Answer from the drawing. Dimensions are ordinates in mm from the lowest x, y and z of the part. A direction names the side the tool comes from. Give positions to 0.01 mm unless a question says otherwise; leave off trailing zeros. Loops run counter-clockwise (first coordinate to the right, second up) from the corner with the lowest first, then second, coordinate; pieces in that order, holes last. Notation, with made-up numbers: (17, -18) - (76, -18) arc R11 ccw to (76, 3) - close; hole circle Ø5 at (28, 10.5). An arc over 180 degrees is marked (long way). Write each question's results on one line, items separated by ' | '. Start each with the question number.
Q1. Given pin 1 (6.5 mm diameter, centred on x = 5, z = 7.5, fed in from +Y); pin 2 (4 mm diameter, centred on y = 2, z = 4, fed in from +X); pin 3 (4 mm diameter, centred on y = 12, z = 7, fed in from -X), each flat-ended and moving along its own axis, determine where each tip first touches the part or whether it passes through.
Q2. The part is cut by section B-B, the plane x = 7.62. Write down the section's boundary in (y, z) (1 decimal).
Q3. Determine the mould class of the marked faces 1, 2, 3 and 4 for opening direction Z: +Z half, -Z half, draft (parallel to the pull), parting line (faces both ways), or undercut.
Q4. The part is cut by section C-C, the plane z = 8.5. State how many separate pieces and enclosed holes the cut face has.
Q5. For the marked faces 5 and 6, determine the directions among +Z, -Z, +X, -X, +Y, -Y from which every point of the face is accessible in a straight line to the end or side of a thin tool.
Q6. Find the intervals of material crossed by line 1 (X direction, y = 13.25, z = 10); line 2 (Z direction, x = 7.62, y = 1.4) (1 decimal); line 3 (Y direction, x = 4, z = 1.5), in increasing order. Write a range as from..to.
Q7. The part is cut by section D-D, the plane y = 7.75. Write down the section's boundary in (x, z).
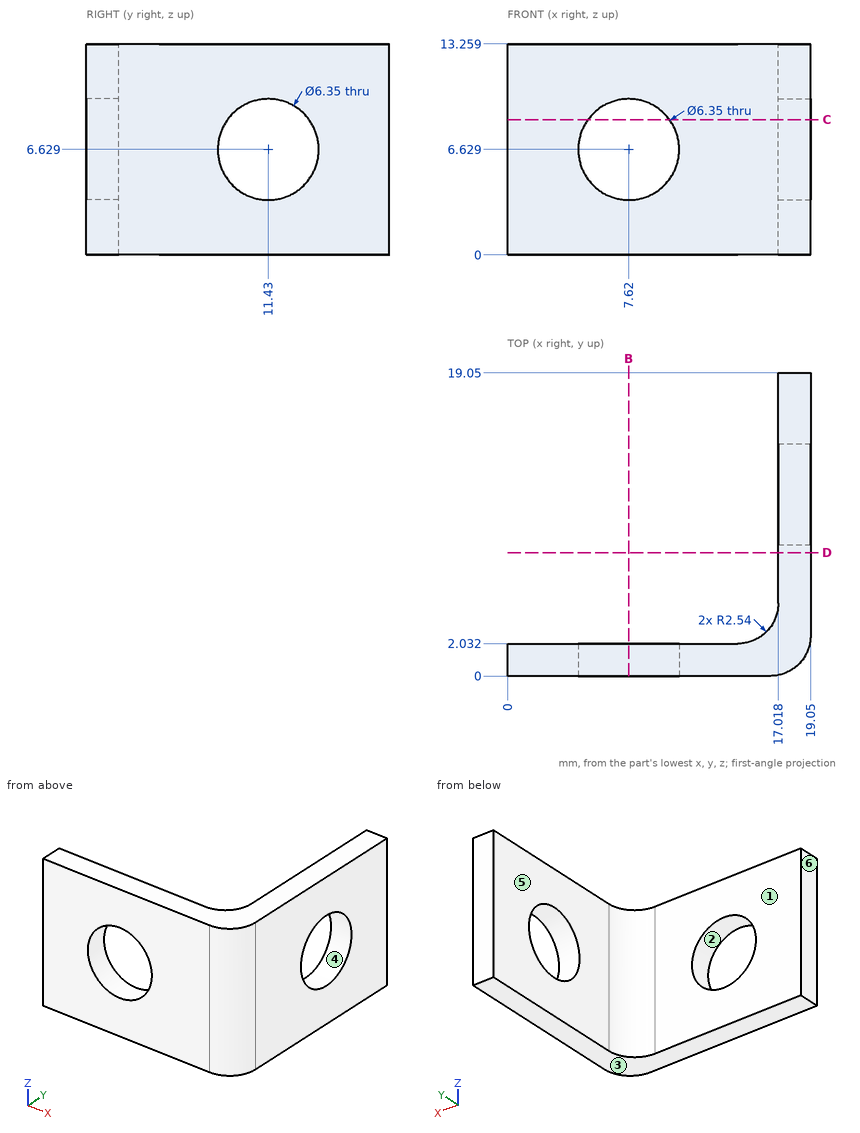
Check sheet entries:
1) pin 1: stops at y = 2.03 | pin 2: stops at x = 19.05 | pin 3: passes through
2) outline: (0, 0) - (2, 0) - (2, 3.5) - (0, 3.5) - close; (0, 9.8) - (2, 9.8) - (2, 13.3) - (0, 13.3) - close
3) face 1: draft | face 2: undercut | face 3: -Z half | face 4: undercut
4) separate pieces: 3 | enclosed holes: 0
5) face 5: +Z, -Z, -X, +Y | face 6: +Z, -Z, -X, +Y, -Y
6) line 1: x = 17.02..19.05 | line 2: z = 0..3.5, 9.8..13.3 | line 3: y = 0..2.03
7) outline: (17.02, 0) - (19.05, 0) - (19.05, 13.26) - (17.02, 13.26) - close
